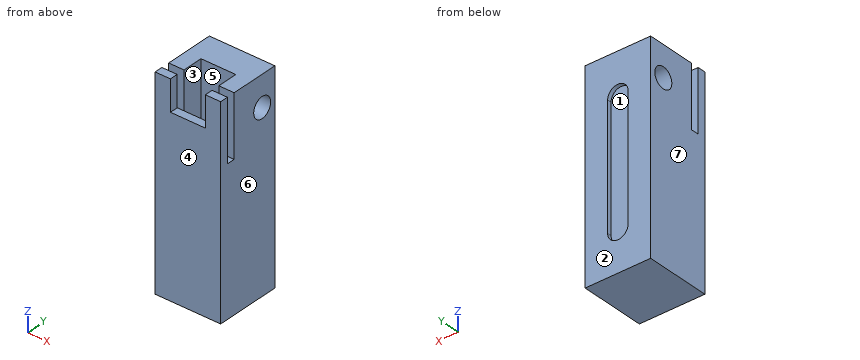
from build123d import *

# Parameters (mm, degrees)
SKETCH1_W               = 32
SKETCH1_H               = 32
BOSS_EXTRUDE1_DEPTH     = 100
CUT_EXTRUDE1_START      = 16
SKETCH2_R               = 5
CUT_EXTRUDE1_DEPTH      = 2
SKETCH3_W               = 17
SKETCH3_H               = 10
CUT_EXTRUDE2_DEPTH      = 30
SKETCH3_4_W             = 8.5
SKETCH3_4_H             = 10.001446171
CUT_EXTRUDE4_DEPTH      = 15
CUT_EXTRUDE3_DEPTH      = 103.528044944
CUT_EXTRUDE3_DEPTH_BACK = 103.528044944
SKETCH4_R               = 5


with BuildPart() as part:
    # Sketch1 → Boss-Extrude1 (new body)
    with BuildSketch(Plane.XY):
        Rectangle(SKETCH1_W, SKETCH1_H)
    extrude(amount=-BOSS_EXTRUDE1_DEPTH)

    # Sketch2 → Cut-Extrude1 (cut)
    with BuildSketch(Plane(origin=(0, 0, 0), x_dir=(1, 0, 0), z_dir=(0, 1, 0)).offset(CUT_EXTRUDE1_START)):
        with BuildLine():
            Line((5, 20), (5, 80))
            ThreePointArc((5, 80), (0, 75), (-5, 80))
            Line((-5, 80), (-5, 20))
            ThreePointArc((-5, 20), (0, 25), (5, 20))
        make_face()
        with Locations((0, 80)):
            Circle(SKETCH2_R)
        with Locations((0, 20)):
            Circle(SKETCH2_R)
    extrude(amount=-CUT_EXTRUDE1_DEPTH, mode=Mode.SUBTRACT)

    # Sketch3 → Cut-Extrude2 (cut)
    with BuildSketch(Plane.XY):
        with Locations((0, -3)):
            Rectangle(SKETCH3_W, SKETCH3_H)
        Polygon((-8.5, -8), (-16, -8), (-16, -12), (-8.5, -12), (8.5, -12), (16, -12), (16, -8), (8.5, -8), align=None)
    extrude(amount=-CUT_EXTRUDE2_DEPTH, mode=Mode.SUBTRACT)

    # Sketch3<4> → Cut-Extrude4 (cut)
    with BuildSketch(Plane.XY):
        with Locations((4.25, -17.000723085)):
            Rectangle(SKETCH3_4_W, SKETCH3_4_H)
        with Locations((-4.25, -17.000723085)):
            Rectangle(SKETCH3_4_W, SKETCH3_4_H)
    extrude(amount=-CUT_EXTRUDE4_DEPTH, mode=Mode.SUBTRACT)

    # Sketch4 → Cut-Extrude3 (cut, two sides: drawn at the far end of the back side and taken through both)
    with BuildSketch(Plane(origin=(0, 0, 0), x_dir=(0, 0, -1), z_dir=(1, 0, 0)).offset(-CUT_EXTRUDE3_DEPTH_BACK)):
        with Locations((15, 8.5)):
            Circle(SKETCH4_R)
    extrude(amount=CUT_EXTRUDE3_DEPTH + CUT_EXTRUDE3_DEPTH_BACK, mode=Mode.SUBTRACT)


solid = part.part
The model under review builds one solid part; all positions refer to its coordinate system, in mm. Face numbers are marked on the shaded views. A direction names the side the tool comes from. Coordinates: 2 decimals unless noted, no trailing zeros. Order: outer loops, then holes, each group sorted by start corner. A loop starts at its lowest first (then second) coordinate and runs counter-clockwise, first axis right, second up. Notation, with made-up numbers: (38.25, 82) -> (49.25, 82) arc R14 cw to (49.25, 109) -> close; hole circle Ø1 at (-39.5, -9.5). An arc over 180 degrees is marked (long way). Answer in a Markdown table with one row per item.
(1) Wall thickness on line 1 along Y through (x, z) = (-6.5, -28); line 2 along X through (y, z) = (14.5, -36.5); line 3 along Z through (x, y) = (4, 8.5): over which ranges is each line inside the solid? List them lowest first.
Answers:
| item | result |
|---|---|
| line 1 | -16 to -12, 2 to 16 |
| line 2 | -16 to -5, 5 to 16 |
| line 3 | -100 to -20, -10 to 0 |
(2) Insertion check: pin 1 (11 mm diameter, centred on x = 0, z = -58, fed in from +Y); pin 2 (6 mm diameter, centred on y = 8.5, z = -15, fed in from -X); pin 3 (1 mm diameter, centred on x = 1, z = -21.5, fed in from +Y); pin 4 (4.5 mm diameter, centred on x = -3, y = -14.5, fed in from +Z). Each pin has a flat end and moves straight along its axis. Give the tip position at first contact, or say it passes through.
Answers:
| item | result |
|---|---|
| pin 1 | y = 16 |
| pin 2 | through |
| pin 3 | y = 14 |
| pin 4 | z = -15 |
(3) Machinability: for the marked faces 1, 2 and 3, which of the approach directions +Z, -Z, +X, -X, +Y, -Y give a long, thin tool a straight path to every point of the face, cutting with its end or side? Answer none if there is none.
Answers:
| item | result |
|---|---|
| face 1 | +Y |
| face 2 | +Z, -Z, +X, -X, +Y |
| face 3 | +Z |
(4) The part is to be moulded in two halves that separate along X. For the marked faces 4, 5, 6 and 7, say which applies: +X half, -X half, draft (parallel to the pull), parting line (faces both ways), or undercut.
Answers:
| item | result |
|---|---|
| face 4 | draft |
| face 5 | undercut |
| face 6 | +X half |
| face 7 | -X half |
(5) Consider section A-A (x = -7). Write out the cut boundary in (y, z).
Answers:
| item | result |
|---|---|
| outline | (-16, -100) -> (16, -100) -> (16, 0) -> (2, 0) -> (2, -30) -> (-12, -30) -> (-12, -15) -> (-16, -15) -> close; hole circle Ø10 at (8.5, -15) |
(6) Consider section B-B (z = -67). Write out the cut boundary in (x, y), plus the area to 3 significant figures.
Answers:
| item | result |
|---|---|
| outline | (-16, -16) -> (16, -16) -> (16, 16) -> (5, 16) -> (5, 14) -> (-5, 14) -> (-5, 16) -> (-16, 16) -> close |
| area | 1,000 mm² |
(7) Consider section C-C (y = 10.5). Write out the cut boundary in (x, z).
Answers:
| item | result |
|---|---|
| outline | (-16, -100) -> (16, -100) -> (16, -19.58) -> (-16, -19.58) -> close; (-16, -10.42) -> (16, -10.42) -> (16, 0) -> (-16, 0) -> close |
(8) Consider section D-D (z = -18.5). Write out the cut boundary in (x, y).
Answers:
| item | result |
|---|---|
| outline | (-16, -16) -> (16, -16) -> (16, -12) -> (-16, -12) -> close; (-16, -8) -> (-8.5, -8) -> (-8.5, 2) -> (8.5, 2) -> (8.5, -8) -> (16, -8) -> (16, 4.93) -> (-16, 4.93) -> close; (-16, 12.07) -> (16, 12.07) -> (16, 16) -> (4.77, 16) -> (4.77, 14) -> (-4.77, 14) -> (-4.77, 16) -> (-16, 16) -> close |
